Read the model definition and answer for the solid it produces. Units are mm, in the model's axes. A direction names the side the tool comes from. Give positions to 0.01 mm unless a question says otherwise; leave off trailing zeros. Loops run counter-clockwise (first coordinate to the right, second up) from the corner with the lowest first, then second, coordinate; pieces in that order, holes last. Notation, with made-up numbers: (54.25, 66) - (90.25, 66) arc R23 cw to (90.25, 99) - close; hole circle Ø2 at (52.25, 33). An arc over 180 degrees is marked (long way). Write item = value, one per line.
```python
from build123d import *

# Parameters (mm, degrees)
F1_DEPTH = 9.398
F2_DEPTH = 9.398
F3_R     = 5.08


with BuildPart() as f1:
    # F0 (on Top) → F1 (new body)
    with BuildSketch(Plane.XY):
        Polygon((-252.907044, 71.313885), (-156.493339, -6.999044), (-150.8083, 0), (-247.171892, 78.272225), align=None)
        with BuildLine():
            Line((-150.8083, 0), (-156.493339, -6.999044))
            ThreePointArc((-156.493339, -6.999044), (-45.311266, 25.097468), (-102.540672, 125.677956))
            Line((-102.540672, 125.677956), (-102.540672, 116.660956))
            ThreePointArc((-102.540672, 116.660956), (-61.639012, 31.42252), (-150.8083, 0))
        make_face()
    extrude(amount=F1_DEPTH)

    # F0 (on Top) → F2 (join)
    with BuildSketch(Plane.XY):
        with BuildLine():
            Line((-150.8083, 0), (-156.493339, -6.999044))
            ThreePointArc((-156.493339, -6.999044), (-45.311266, 25.097468), (-102.540672, 125.677956))
            Line((-102.540672, 125.677956), (-102.540672, 116.660956))
            ThreePointArc((-102.540672, 116.660956), (-61.639012, 31.42252), (-150.8083, 0))
        make_face()
        Polygon((-252.907044, 71.313885), (-156.493339, -6.999044), (-150.8083, 0), (-247.171892, 78.272225), align=None)
        Polygon((-267.090976, 87.734386), (-252.907044, 71.313885), (-247.171892, 78.272225), (-257.171273, 89.76128), (-249.178657, 96.717571), (-253.950546, 102.200361), align=None)
    extrude(amount=F2_DEPTH)

    # F3
    f3_edges = [f1.edges().sort_by_distance(p)[0] for p in [
        (-267.090976, 87.734386, 4.699),
    ]]
    fillet(f3_edges, radius=F3_R)


solid = f1.part
```
1) Each of these flat-tipped pins is pushed along its axis until it touches: P1, Ø2.5, axis at y = 120.5, z = 5.5, coming from the -X side; P2, Ø3, axis at x = -150.5, z = 2, coming from the -Y side; P3, Ø8, axis at x = -209, y = 48.5, coming from the -Z side. Where does it stop, or does it pass through?
Output:
P1 = -102.54
P2 = -11.72
P3 = 0
2) Find the intervals of material crossed by probe 1 along X at (y, z) = (72, 6.25); probe 2 along X at (y, z) = (58, 1.75); probe 3 along Y at (x, z) = (-65, 8), in increasing order.
Output:
probe_1 = -253.5 to -239.45, -58.94 to -42.42
probe_2 = -236.52 to -222.21, -56.86 to -40.07
probe_3 = -2.56 to 24.51, 86.88 to 108.24
3) A cutting plane is placed at D-D on x = -134.5. Determine the outline of the cut face in (y, z), then the cut area to 3 significant figures.
Output:
outline = (-17.77, 0) - (-6.2, 0) - (-6.2, 9.4) - (-17.77, 9.4) - close
area = 109 mm²
4) A tool of negligible diameter and unlimited length cuts with its end or side. For faces 5 (the face through (-198.32, 38.59, 4.63)), 6 (the face through (-205.38, 32.71, 4.63)), 7 (the face through (-252.102, 83.936, 4.633)), from which of +Z, -Z, +X, -X, +Y, -Y can it reach the whole face along a straight path? Write none if from no direction.
Output:
face_5 = +Z, -Z, +Y
face_6 = +Z, -Z, -X, -Y
face_7 = +Z, -Z
5) A cutting plane is placed at C-C on z = 4.25. Determine the outline of the cut face in (x, y) (3 decimals).
Output:
outline = (-264.149, 84.329) - (-252.907, 71.314) - (-156.493, -6.999) arc R73.66 ccw (long way) to (-102.541, 125.678) - (-102.541, 116.661) arc R63.5 cw (long way) to (-150.808, 0) - (-247.172, 78.272) - (-257.171, 89.761) - (-249.179, 96.718) - (-253.951, 102.2) - (-264.065, 91.065) arc R5.08 ccw to start
6) The mould has two halves that part along Y. Classify faces 1 (the face through (-251.53, 99.42, 4.63)), 2 (the face through (-102.541, 121, 5)), 3 (the face through (-258.607, 77.913, 4.633)), 4 (the face through (-61.084, 32.809, 4.633)): pulls with the +Y half, pulls with the -Y half, needs draft (parallel to the pull), parting line crosses it, or undercut.
Output:
face_1 = pulls with the +Y half
face_2 = needs draft
face_3 = pulls with the -Y half
face_4 = undercut
7) A cutting plane is placed at A-A on x = -76. Determine the outline of the cut face in (y, z).
Output:
outline = (-10.53, 0) - (10.22, 0) - (10.22, 9.4) - (-10.53, 9.4) - close; (101.18, 0) - (116.22, 0) - (116.22, 9.4) - (101.18, 9.4) - close
8) A cutting plane is placed at B-B on y = 36. Determine the outline of the cut face in (x, z).
Output:
outline = (-209.43, 0) - (-195.13, 0) - (-195.13, 9.4) - (-209.43, 9.4) - close; (-59.95, 0) - (-41.84, 0) - (-41.84, 9.4) - (-59.95, 9.4) - close
